The drawing under review shows one solid part. Ordinate dimensions are in mm from its lowest x, y, z. A direction names the side the tool comes from. Give positions to 0.01 mm unless a question says otherwise; leave off trailing zeros. Loops run counter-clockwise (first coordinate to the right, second up) from the corner with the lowest first, then second, coordinate; pieces in that order, holes last. Notation, with made-up numbers: (72, 88.25) - (96, 88.25) arc R18 cw to (96, 108.25) - close; hole circle Ø6 at (35, 19). An arc over 180 degrees is marked (long way). Answer as CSV lines item,"result".
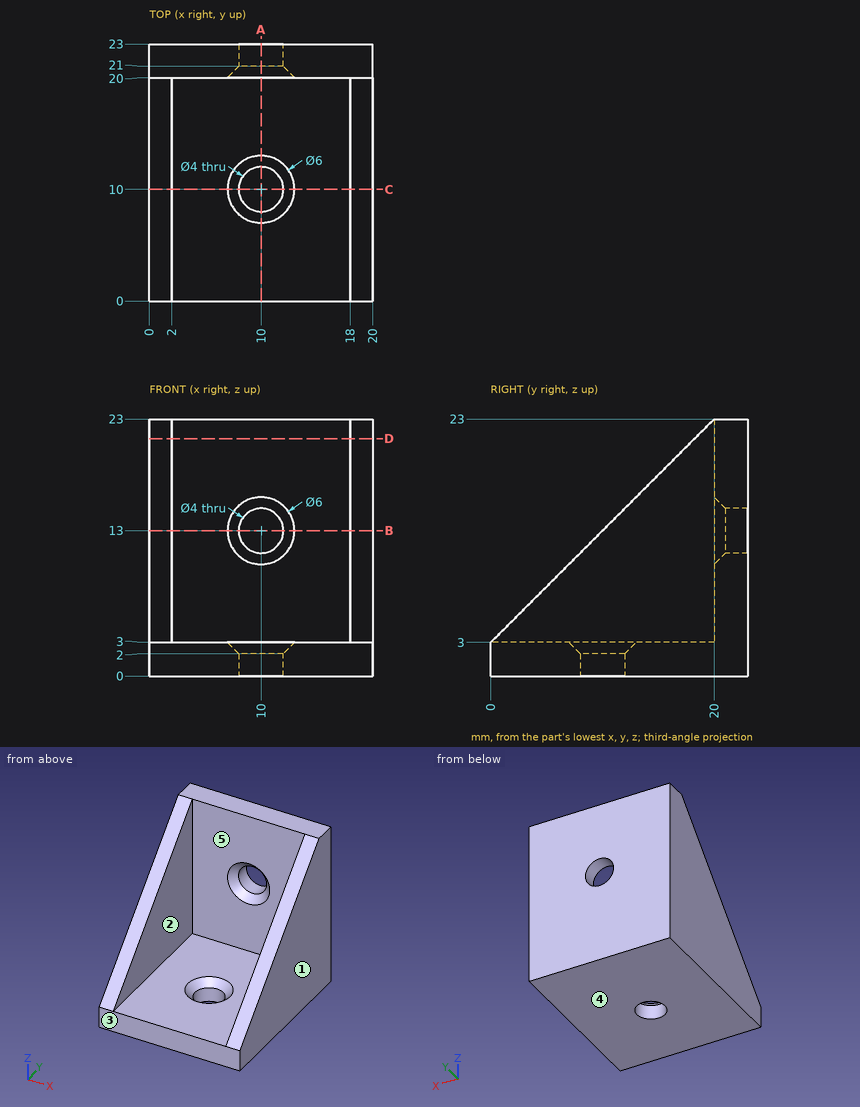
1) Insertion check: P1, Ø5, axis at x = 10, z = 13, coming from the -Y side; P2, Ø8, axis at x = 10, z = 18, coming from the -Y side; P3, Ø5, axis at x = 8.5, y = 4.5, coming from the +Z side; P4, Ø2.5, axis at x = 10, y = 10, coming from the +Z side. Each pin has a flat end and moves straight along its axis. Give the tip position at first contact, or say it passes through.
From the geometry:
P1,"stops at y = 20.5"
P2,"stops at y = 20"
P3,"stops at z = 3"
P4,"passes through"
2) Machinability: for the marked faces 4 and 5, which of the approach directions +Z, -Z, +X, -X, +Y, -Y give a long, thin tool a straight path to every point of the face, cutting with its end or side? Answer none if there is none.
From the geometry:
face 4,"-Z, +X, -X, +Y, -Y"
face 5,"+Z, -Y"
3) Consider section B-B on z = 13. Write out the cut boundary in (x, y).
From the geometry:
outline,"(0, 10) - (2, 10) - (2, 20) - (7, 20) - (8, 21) - (8, 23) - (0, 23) - close; (12, 21) - (13, 20) - (18, 20) - (18, 10) - (20, 10) - (20, 23) - (12, 23) - close"
4) Consider section D-D on z = 21.25. Write out the cut boundary in (x, y), and give its area (3 significant figures).
From the geometry:
outline,"(0, 18.25) - (2, 18.25) - (2, 20) - (18, 20) - (18, 18.25) - (20, 18.25) - (20, 23) - (0, 23) - close"
area,"67.0 mm^2"
5) Draft analysis for pull direction X (two halves, no side actions). For the marked faces 1, 2 and 3, state which applies: pulls with the +X half, pulls with the -X half, needs draft (parallel to the pull), parting line crosses it, or undercut.
From the geometry:
face 1,"pulls with the +X half"
face 2,"undercut"
face 3,"needs draft"
6) Consider section C-C on y = 10. Write out the cut boundary in (x, z).
From the geometry:
outline,"(0, 0) - (8, 0) - (8, 2) - (7, 3) - (2, 3) - (2, 13) - (0, 13) - close; (12, 0) - (20, 0) - (20, 13) - (18, 13) - (18, 3) - (13, 3) - (12, 2) - close"
7) Wall thickness on line 1 (Y direction, x = 10, z = 1); line 2 (X direction, y = 8.75, z = 9.75); line 3 (Z direction, x = 10, y = 21.8): over which ranges is each line inside the solid? List them lowest first. Write a range as from..to.
From the geometry:
line 1,"y = 0..8, 12..23"
line 2,"x = 0..2, 18..20"
line 3,"z = 0..11, 15..23"
8) Consider section A-A on x = 10. Write out the cut boundary in (y, z), and give its area (3 significant figures).
From the geometry:
outline,"(0, 0) - (8, 0) - (8, 2) - (7, 3) - (0, 3) - close; (12, 0) - (23, 0) - (23, 11) - (21, 11) - (20, 10) - (20, 3) - (13, 3) - (12, 2) - close; (20, 16) - (21, 15) - (23, 15) - (23, 23) - (20, 23) - close"
area,"103 mm^2"
